Could you check a few things on this drawing? It's one solid part, dimensions in mm from its lowest x, y, z. Coordinates: 2 decimals unless noted, no trailing zeros. Write each loop counter-clockwise with the first axis right and the second up, starting at its lowest first coordinate (ties: lowest second). Pieces come first, ordered by that corner, then holes. Notation, with made-up numbers: (29, 67) - (57, 67) arc R30 ccw to (57, 102) - close; hole circle Ø8 at (75, -39). An arc over 180 degrees is marked (long way). Answer as a JSON object with one key per item and string values. Group by question number.
1) If we section it at D-D (x = 2.75): Write out the boundary of the cut face in (y, z), plus the area to 3 significant figures.
2) If we section it at C-C (z = 20.5): Write out the boundary of the cut face in (x, y).
3) If we section it at A-A (x = 6): Write out the boundary of the cut face in (y, z).
4) Please list where these lines run through material, in increasing order: line 1 along Y through (x, z) = (6, 16.5); line 2 along Z through (x, y) = (9, 9.25); line 3 along X through (y, z) = (8.5, 33.5).
5) We'd pull the mould along X, two halves only. Please class the marked faces 1, 2 and 3: released by +X, released by -X, zero draft, split by the parting line, or undercut.
6) If we section it at B-B (y = 6.5): Write out the boundary of the cut face in (x, z).
7) Will these pins go through, and if not, where does the flat tip stop? pin 1 Ø1 at (x, z) = (7.5, 21) entering from -Y; pin 2 Ø6 at (y, z) = (2, 15) entering from -X; pin 3 Ø6 at (x, z) = (6.5, 4.5) entering from +Y.
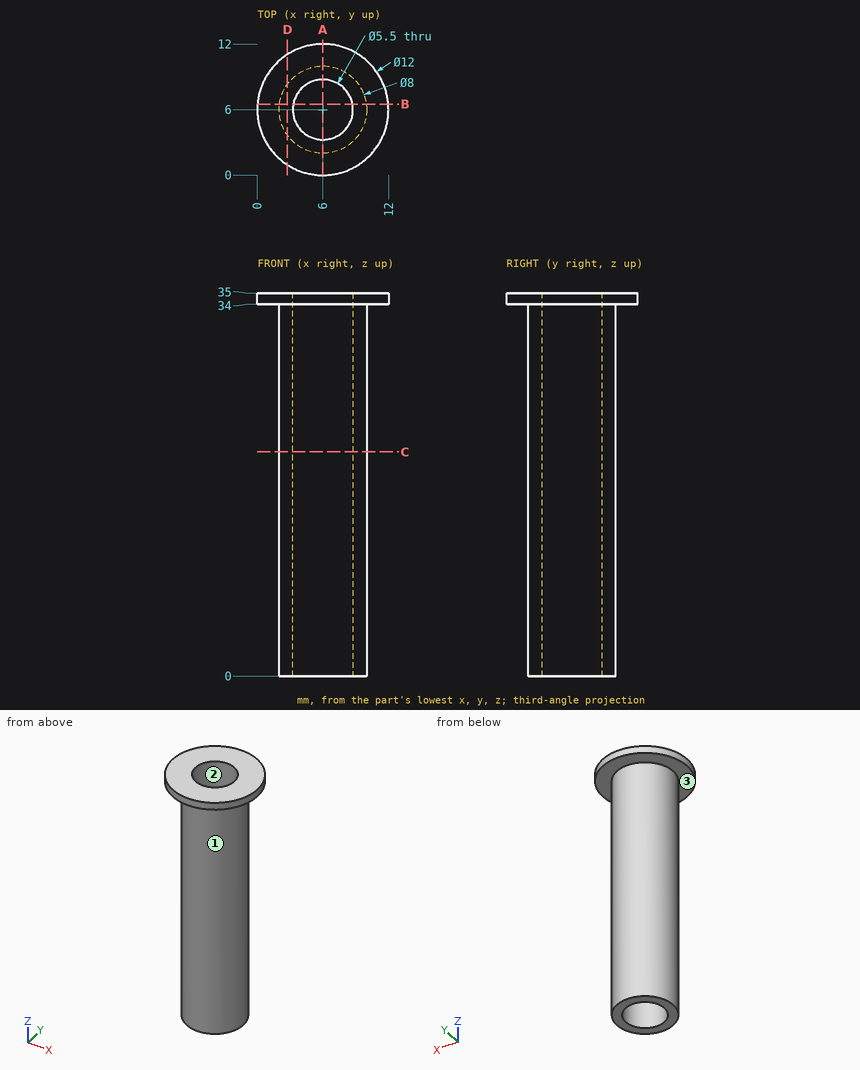
Here are the results:
{
 "1": {"outline": "(0.96, 34) - (3.67, 34) - (3.67, 0) - (8.33, 0) - (8.33, 34) - (11.04, 34) - (11.04, 35) - (0.96, 35) - close", "area": "169 mm²"},
 "2": {"outline": "circle Ø8 at (6, 6); hole circle Ø5.5 at (6, 6)"},
 "3": {"outline": "(0, 34) - (2, 34) - (2, 0) - (3.25, 0) - (3.25, 35) - (0, 35) - close; (8.75, 0) - (10, 0) - (10, 34) - (12, 34) - (12, 35) - (8.75, 35) - close"},
 "4": {"line 1": "y = 2 to 3.25, 8.75 to 10", "line 2": "z = 34 to 35", "line 3": "x = 2.88 to 4.85, 7.15 to 9.12"},
 "5": {"face 1": "split by the parting line", "face 2": "undercut", "face 3": "zero draft"},
 "6": {"outline": "(0.02, 34) - (2.03, 34) - (2.03, 0) - (3.3, 0) - (3.3, 35) - (0.02, 35) - close; (8.7, 0) - (9.97, 0) - (9.97, 34) - (11.98, 34) - (11.98, 35) - (8.7, 35) - close"},
 "7": {"pin 1": "stops at y = 2.13", "pin 2": "stops at x = 2.13", "pin 3": "stops at y = 10"}
}
